```python
from build123d import *
from build123d.topology import SkipClean

# Parameters (mm, degrees)
SKETCH_1_R          = 9.5
EXTRUDE_1_DEPTH     = 4
SKETCH_2_W          = 20
SKETCH_2_H          = 30
EXTRUDE_2_DEPTH     = 4
CUT_EXTRUDE_START   = -4
CUT_EXTRUDE_1_DEPTH = 4
EXTRUDE_3_DEPTH     = 4
CUT_EXTRUDE_2_DEPTH = 4
SKETCH_6_R          = 2
CUT_EXTRUDE_3_DEPTH = 4
FILLET_1_R          = 2


with BuildPart() as part:
    # 草图1 → 凸台-拉伸1 (new body)
    with BuildSketch(Plane.XY):
        with BuildLine():
            Line((-16.5, 0), (-16.5, 73))
            Line((-16.5, 73), (16.5, 73))
            Line((16.5, 73), (16.5, 0))
            ThreePointArc((16.5, 0), (0, -16.5), (-16.5, 0))
        make_face()
        Circle(SKETCH_1_R, mode=Mode.SUBTRACT)
    extrude(amount=EXTRUDE_1_DEPTH)

    # 草图2 → 凸台-拉伸2 (add)
    with BuildSketch(Plane.XY.offset(4)):
        with Locations((26.5, 58)):
            Rectangle(SKETCH_2_W, SKETCH_2_H)
    extrude(amount=-EXTRUDE_2_DEPTH)

    # 草图3 → 切除-拉伸1 (cut)
    with BuildSketch(Plane.XY.offset(4).offset(CUT_EXTRUDE_START)):
        with BuildLine():
            Line((-15.707266889, 5.052896881), (-3.5, 43))
            Line((-3.5, 43), (-3.5, 73))
            Line((-3.5, 73), (-16.5, 73))
            Line((-16.5, 73), (-16.5, 0))
            ThreePointArc((-16.5, 0), (-16.300612008, 2.557351788), (-15.707266889, 5.052896881))
        make_face()
    extrude(amount=CUT_EXTRUDE_1_DEPTH, mode=Mode.SUBTRACT)

    # 草图4 → 凸台-拉伸3 (add)
    with BuildSketch(Plane(origin=(0, 0, 0), x_dir=(-1, 0, 0), z_dir=(0, 0, -1))):
        Polygon((-36.5, 43), (-15.152569354, -6.530669335), (-9.5, 0), (-16.5, 43), align=None)
    extrude(amount=-EXTRUDE_3_DEPTH)

    # 草图5 → 切除-拉伸2 (cut)
    with SkipClean():  # the faces are left unmerged after this step: merging them gives an invalid solid
        with BuildSketch(Plane.XY.offset(4).offset(CUT_EXTRUDE_START)):
            with BuildLine():
                Line((-3.5, 43), (-3.5, 33))
                ThreePointArc((-3.5, 33), (-5.718901629, 21.313506702), (-12.066772655, 11.253577107))
                ThreePointArc((-12.066772655, 11.253577107), (-14.228894088, 8.353955533), (-15.707266889, 5.052896881))
                Line((-15.707266889, 5.052896881), (-3.5, 43))
            make_face()
        extrude(amount=CUT_EXTRUDE_2_DEPTH, mode=Mode.SUBTRACT)

    # 草图6 → 切除-拉伸3 (cut)
    with SkipClean():  # the faces are left unmerged after this step: merging them gives an invalid solid
        with BuildSketch(Plane(origin=(0, 0, 0), x_dir=(-1, 0, 0), z_dir=(0, 0, -1))):
            with Locations((-31.5, 67.5)):
                Circle(SKETCH_6_R)
            with Locations((-1.5, 67.5)):
                Circle(SKETCH_6_R)
            with Locations((-31.5, 48.5)):
                Circle(SKETCH_6_R)
            with Locations((-1.5, 48.5)):
                Circle(SKETCH_6_R)
        extrude(amount=-CUT_EXTRUDE_3_DEPTH, mode=Mode.SUBTRACT)

    # 圆角1
    fillet_1_edges = [part.edges().sort_by_distance(p)[0] for p in [
        (36.5, 73, 2),
        (36.5, 43, 2),
        (-3.5, 73, 2),
    ]]
    fillet(fillet_1_edges, radius=FILLET_1_R)


solid = part.part
```
Here's how the part is built. I have some questions about the finished solid (model axes, mm). Round coordinates to 2 decimals unless told otherwise and drop trailing zeros. Order: outer loops, then holes, each group sorted by start corner. A loop starts at its lowest first (then second) coordinate and runs counter-clockwise, first axis right, second up. Notation, with made-up numbers: (-17, 63.25) -> (31, 63.25) arc R18 ccw to (31, 78.25) -> close; hole circle Ø2 at (-10.5, 39.5). An arc over 180 degrees is marked (long way). Use a Markdown table: item, result. Add a question column.
(1) I need wall thicknesses on line 1 along Y through (x, z) = (32, 3.6); line 2 along Y through (x, z) = (31.5, 2.6); line 3 along Y through (x, z) = (1, 1.25). Which ranges of each line are inside material? Lowest first, please.
(2) Suppose I cut it at A-A, the plane z = 2.45. Please give me the cut outline in (x, y).
(3) Suppose I cut it at C-C, the plane y = 67.5. Please give me the cut outline in (x, z), and give its area (3 significant figures).
(4) Suppose I cut it at D-D, the plane x = -6.5. Please give me the cut outline in (y, z).
(5) If we mould it in two halves opening along X, with no side actions, what happens to faces 1 (the face through (10, 39, 0)), 2 (the face through (-3.5, 52, 2)), 3 (the face through (1.76, 69.483, 1.972))? For each: released by +X, released by -X, zero draft, split by the parting line, or undercut.
(6) Suppose I cut it at B-B, the plane x = 1.5. Please give me the cut outline in (y, z), and give its area (3 significant figures).
Verdict:
| question | item | result |
|---|---|---|
| 1 | line 1 | 32.56 to 46.56, 50.44 to 65.56, 69.44 to 73 |
| 1 | line 2 | 31.4 to 46.5, 50.5 to 65.5, 69.5 to 73 |
| 1 | line 3 | -16.47 to -9.45, 9.45 to 46.56, 50.44 to 65.56, 69.44 to 73 |
| 2 | outline | (-12.07, 11.25) arc R16.5 ccw (long way) to (15.15, -6.53) -> (36.34, 42.62) arc R2 ccw to (36.5, 43.41) -> (36.5, 71) arc R2 ccw to (34.5, 73) -> (-1.5, 73) arc R2 ccw to (-3.5, 71) -> (-3.5, 33) arc R31.88 cw to start; hole circle Ø19 at (0, 0); hole circle Ø4 at (1.5, 48.5); hole circle Ø4 at (1.5, 67.5); hole circle Ø4 at (31.5, 48.5); hole circle Ø4 at (31.5, 67.5) |
| 3 | outline | (-3.5, 0) -> (-0.5, 0) -> (-0.5, 4) -> (-3.5, 4) -> close; (3.5, 0) -> (29.5, 0) -> (29.5, 4) -> (3.5, 4) -> close; (33.5, 0) -> (36.5, 0) -> (36.5, 4) -> (33.5, 4) -> close |
| 3 | area | 128 mm2 |
| 4 | outline | (-15.17, 0) -> (-6.93, 0) -> (-6.93, 4) -> (-15.17, 4) -> close; (6.93, 0) -> (19.5, 0) -> (19.5, 4) -> (6.93, 4) -> close |
| 5 | face 1 | zero draft |
| 5 | face 2 | released by -X |
| 5 | face 3 | undercut |
| 6 | outline | (-16.43, 0) -> (-9.38, 0) -> (-9.38, 4) -> (-16.43, 4) -> close; (9.38, 0) -> (46.5, 0) -> (46.5, 4) -> (9.38, 4) -> close; (50.5, 0) -> (65.5, 0) -> (65.5, 4) -> (50.5, 4) -> close; (69.5, 0) -> (73, 0) -> (73, 4) -> (69.5, 4) -> close |
| 6 | area | 251 mm2 |
